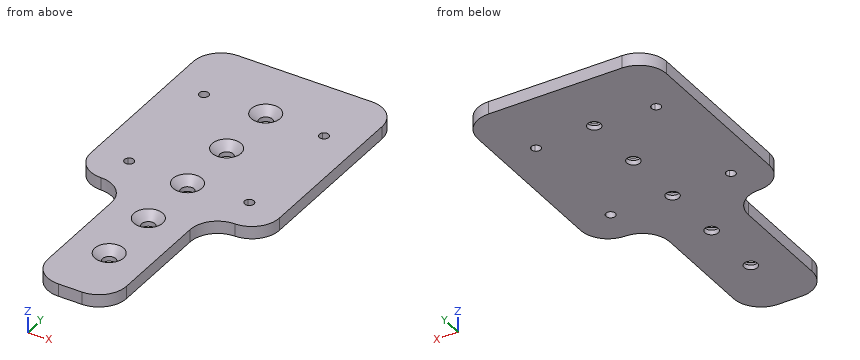
from build123d import *

# Parameters (mm, degrees)
F0_W     = 60
F0_H     = 160
F1_DEPTH = 4
F2_W     = 60
F2_H     = 40
F3_DEPTH = 4.001
F4_R     = 2.1
F5_DEPTH = 4.001
F6_SIZE  = 2.5
F7_W     = 17.5
F7_H     = 50
F8_DEPTH = 4.001
F9_R     = 8.74999


# Not quite as in the source:
# - a fillet or chamfer is up to 0.001 mm smaller than in the source, because OpenCascade refuses the exact size


with BuildPart() as f1:
    # F0 (on Top) → F1 (new body)
    with BuildSketch(Plane.XY):
        Rectangle(F0_W, F0_H)
        with BuildLine():
            ThreePointArc((20.122671197, 18.002169422), (25.2221343498, 9.6355559695), (27, 0))
            ThreePointArc((27, 0), (25.2221343498, -9.6355559695), (20.122671197, -18.002169422))
            ThreePointArc((20.122671197, -18.002169422), (20.4695953547, -18.4986639746), (20.591883092, -19.091883092))
            ThreePointArc((20.591883092, -19.091883092), (19.6466035148, -20.4855420362), (18.002169422, -20.122671197))
            ThreePointArc((18.002169422, -20.122671197), (0, -27), (-18.002169422, -20.122671197))
            ThreePointArc((-18.002169422, -20.122671197), (-20.1525432638, -20.1525432638), (-20.122671197, -18.002169422))
            ThreePointArc((-20.122671197, -18.002169422), (-27, 0), (-20.122671197, 18.002169422))
            ThreePointArc((-20.122671197, 18.002169422), (-20.1525432638, 20.1525432638), (-18.002169422, 20.122671197))
            ThreePointArc((-18.002169422, 20.122671197), (0, 27), (18.002169422, 20.122671197))
            ThreePointArc((18.002169422, 20.122671197), (19.6466035148, 20.4855420362), (20.591883092, 19.091883092))
            ThreePointArc((20.591883092, 19.091883092), (20.4695953547, 18.4986639746), (20.122671197, 18.002169422))
        make_face(mode=Mode.SUBTRACT)
        with BuildLine():
            Line((-18.0312229203, -18.0312229203), (0, 0))
            Line((0, 0), (-18.0312229203, 18.0312229203))
            ThreePointArc((-18.0312229203, 18.0312229203), (-19.0710477486, 17.5920278029), (-20.122671197, 18.002169422))
            ThreePointArc((-20.122671197, 18.002169422), (-27, 0), (-20.122671197, -18.002169422))
            ThreePointArc((-20.122671197, -18.002169422), (-19.0710477486, -17.5920278029), (-18.0312229203, -18.0312229203))
        make_face()
        with BuildLine():
            Line((0, 0), (18.0312229203, 18.0312229203))
            ThreePointArc((18.0312229203, 18.0312229203), (17.5920278029, 19.0710477486), (18.002169422, 20.122671197))
            ThreePointArc((18.002169422, 20.122671197), (0, 27), (-18.002169422, 20.122671197))
            ThreePointArc((-18.002169422, 20.122671197), (-17.6982241479, 19.6466035148), (-17.591883092, 19.091883092))
            ThreePointArc((-17.591883092, 19.091883092), (-17.7060637933, 18.5178579435), (-18.0312229203, 18.0312229203))
            Line((-18.0312229203, 18.0312229203), (0, 0))
        make_face()
        with BuildLine():
            ThreePointArc((20.122671197, -18.002169422), (25.2221343498, -9.6355559695), (27, 0))
            ThreePointArc((27, 0), (25.2221343498, 9.6355559695), (20.122671197, 18.002169422))
            ThreePointArc((20.122671197, 18.002169422), (19.0710477486, 17.5920278029), (18.0312229203, 18.0312229203))
            Line((18.0312229203, 18.0312229203), (0, 0))
            Line((0, 0), (18.0312229203, -18.0312229203))
            ThreePointArc((18.0312229203, -18.0312229203), (19.0710477486, -17.5920278029), (20.122671197, -18.002169422))
        make_face()
        with BuildLine():
            ThreePointArc((18.002169422, -20.122671197), (17.5920278029, -19.0710477486), (18.0312229203, -18.0312229203))
            Line((18.0312229203, -18.0312229203), (0, 0))
            Line((0, 0), (-18.0312229203, -18.0312229203))
            ThreePointArc((-18.0312229203, -18.0312229203), (-17.7060637933, -18.5178579435), (-17.591883092, -19.091883092))
            ThreePointArc((-17.591883092, -19.091883092), (-17.6982241479, -19.6466035148), (-18.002169422, -20.122671197))
            ThreePointArc((-18.002169422, -20.122671197), (0, -27), (18.002169422, -20.122671197))
        make_face()
    extrude(amount=F1_DEPTH)

    # F2 (on face) → F3 (cut, through all)
    with BuildSketch(Plane.XY.offset(4)):
        with Locations((0, 60)):
            Rectangle(F2_W, F2_H)
    extrude(amount=-F3_DEPTH, mode=Mode.SUBTRACT)

    # F4 (on face) → F5 (cut, through all)
    with BuildSketch(Plane(origin=(0, 0, 0), x_dir=(1, 0, 0), z_dir=(0, 0, -1))):
        with Locations((0, 40)):
            Circle(F4_R)
        Circle(F4_R)
        with Locations((0, 20)):
            Circle(F4_R)
        with Locations((0, -20)):
            Circle(F4_R)
        with Locations((0, 60)):
            Circle(F4_R)
    extrude(amount=-F5_DEPTH, mode=Mode.SUBTRACT)

    # F6
    f6_edges = [f1.edges().sort_by_distance(p)[0] for p in [
        (-2.1, -60, 4),
        (-2.1, -40, 4),
        (-2.1, -20, 4),
        (-2.1, 0, 4),
        (-2.1, 20, 4),
    ]]
    chamfer(f6_edges, length=F6_SIZE)

    # F7 (on face) → F8 (cut, through all)
    with BuildSketch(Plane(origin=(0, 0, 0), x_dir=(1, 0, 0), z_dir=(0, 0, -1))):
        with Locations((-21.25, 55)):
            Rectangle(F7_W, F7_H)
        with Locations((21.25, 55)):
            Rectangle(F7_W, F7_H)
    extrude(amount=-F8_DEPTH, mode=Mode.SUBTRACT)

    # F9 (radius 8.75 in the source; OpenCascade refuses exactly that, so slightly less here)
    f9_edges = [f1.edges().sort_by_distance(p)[0] for p in [
        (-12.5, -30, 2),
        (-30, -30, 2),
        (12.5, -30, 2),
        (30, -30, 2),
        (-30, 40, 2),
        (30, 40, 2),
        (-12.5, -80, 2),
        (12.5, -80, 2),
    ]]
    fillet(f9_edges, radius=F9_R)


solid = f1.part
Model file for the job. Use its own axes, mm. Round coordinates to 2 decimals unless told otherwise and drop trailing zeros. Order: outer loops, then holes, each group sorted by start corner. A loop starts at its lowest first (then second) coordinate and runs counter-clockwise, first axis right, second up. Notation, with made-up numbers: M 43.25,46.5 L 57.25,46.5 A16 cw 57.25,75.5 Z; hole C 55,-38.75 d4. An arc over 180 degrees is marked long. Write each question's results on one line, items separated by ' | '. Start each with the question number.
(1) Probe probe 1 along Y at (x, z) = (0, 1.1); probe 2 along X at (y, z) = (0, 0.4); probe 3 along X at (y, z) = (-20, 0.7). List the from-to ranges inside material, lowest first. Write a range as from..to.
(2) Saw through at C-C, the plane y = 0. Give the cut face in (x, z), then the cut area to 3 significant figures.
(3) Drop flat-ended pins along their axis: pin 1 (1 mm diameter, centred on y = -40.5, z = 3.5, fed in from +X); pin 2 (1.2 mm diameter, centred on y = -54, z = 2.5, fed in from -X); pin 3 (6.5 mm diameter, centred on x = 0, y = -60, fed in from +Z). Give the stop position or say it passes through.
(4) Saw through at B-B, the plane x = 0. State how many separate pieces and enclosed holes the cut face has, then the cut area to 3 significant figures.
(5) Saw through at A-A, the plane y = -40. Give the cut face in (x, z), then the cut area to 4 significant figures.
Established:
1) probe 1: y = -80..-62.1, -57.9..-42.1, -37.9..-22.1, -17.9..-2.1, 2.1..17.9, 22.1..40 | probe 2: x = -30..-2.1, 2.1..30 | probe 3: x = -30..-20.29, -17.9..-2.1, 2.1..17.9, 20.29..30
2) outline: M -30,0 L -2.1,0 L -2.1,1.5 L -4.6,4 L -30,4 Z; M 2.1,0 L 30,0 L 30,4 L 4.6,4 L 2.1,1.5 Z | area: 217 mm^2
3) pin 1: stops at x = 12.5 | pin 2: stops at x = -12.5 | pin 3: stops at z = 2.65
4) separate pieces: 6 | enclosed holes: 0 | area: 365 mm^2
5) outline: M -12.5,0 L -2.1,0 L -2.1,1.5 L -4.6,4 L -12.5,4 Z; M 2.1,0 L 12.5,0 L 12.5,4 L 4.6,4 L 2.1,1.5 Z | area: 76.95 mm^2
